```python
from build123d import *

# Parameters (mm, degrees)
SKETCH1_R           = 40.5
SKETCH1_R_2         = 1.75
SKETCH1_R_3         = 33.75
BOSS_EXTRUDE1_DEPTH = 15.5
SKETCH2_R           = 0.75
CUT_EXTRUDE1_DEPTH  = 60.335908184


with BuildPart() as part:
    # Sketch1 → Boss-Extrude1 (new body)
    with BuildSketch(Plane(origin=(0, 0, 0), x_dir=(1, 0, 0), z_dir=(0, 1, 0))):
        with Locations(Location((0, 0, 0), (0, 0, 270))):
            Circle(SKETCH1_R)
        with Locations(Location((0, 37.25, 0), (0, 0, 270))):
            Circle(SKETCH1_R_2, mode=Mode.SUBTRACT)
        with Locations(Location((21.895000648, 30.13588304, 0), (0, 0, 270))):
            Circle(SKETCH1_R_2, mode=Mode.SUBTRACT)
        with Locations(Location((35.426855232, 11.51088304, 0), (0, 0, 270))):
            Circle(SKETCH1_R_2, mode=Mode.SUBTRACT)
        with Locations(Location((35.426855232, -11.51088304, 0), (0, 0, 270))):
            Circle(SKETCH1_R_2, mode=Mode.SUBTRACT)
        with Locations(Location((21.895000648, -30.13588304, 0), (0, 0, 270))):
            Circle(SKETCH1_R_2, mode=Mode.SUBTRACT)
        with Locations(Location((0, -37.25, 0), (0, 0, 270))):
            Circle(SKETCH1_R_2, mode=Mode.SUBTRACT)
        with Locations(Location((-21.895000648, -30.13588304, 0), (0, 0, 270))):
            Circle(SKETCH1_R_2, mode=Mode.SUBTRACT)
        with Locations(Location((-35.426855232, -11.51088304, 0), (0, 0, 270))):
            Circle(SKETCH1_R_2, mode=Mode.SUBTRACT)
        with Locations(Location((-35.426855232, 11.51088304, 0), (0, 0, 270))):
            Circle(SKETCH1_R_2, mode=Mode.SUBTRACT)
        with Locations(Location((-21.895000648, 30.13588304, 0), (0, 0, 270))):
            Circle(SKETCH1_R_2, mode=Mode.SUBTRACT)
        with Locations(Location((0, 0, 0), (0, 0, 270))):
            Circle(SKETCH1_R_3, mode=Mode.SUBTRACT)
    extrude(amount=BOSS_EXTRUDE1_DEPTH)

    # Sketch2 → Cut-Extrude1 (cut, through all)
    with BuildSketch(Plane(origin=(0, 15.5, 0), x_dir=(1, 0, 0), z_dir=(0, 1, 0))):
        with Locations(Location((-6.483486619, -35.325442924, 0), (0, 0, 270))):
            Circle(SKETCH2_R)
        with Locations(Location((-15.518523524, -32.389781477, 0), (0, 0, 270))):
            Circle(SKETCH2_R)
    extrude(amount=-CUT_EXTRUDE1_DEPTH, mode=Mode.SUBTRACT)


solid = part.part
```
Geometry check sheet. Reference: the model listing, model coordinates, mm. Coordinates: 2 decimals unless noted, no trailing zeros. Order: outer loops, then holes, each group sorted by start corner. A loop starts at its lowest first (then second) coordinate and runs counter-clockwise, first axis right, second up.
Q1. Depth check by flat-ended pin: pin 1 Ø4 at (y, z) = (4.5, -11) entering from +X; pin 2 Ø5 at (y, z) = (13, 23.5) entering from +X; pin 3 Ø2 at (x, y) = (24, 5) entering from -Z. Enter the tip coordinate at first touch or a pass-through.
Reply:
pin 1: stops at x = 39.49
pin 2: stops at x = 34.63
pin 3: stops at z = -33.34
Q2. Thickness scan on probe 1 along Z at (x, y) = (23, 3.75); probe 2 along X at (y, z) = (6.5, 0); probe 3 along X at (y, z) = (9, 10). Record the ranges inside material, lowest first.
Reply:
probe 1: z = -33.34 to -31.49, -28.78 to -24.7, 24.7 to 28.78, 31.49 to 33.34
probe 2: x = -40.5 to -33.75, 33.75 to 40.5
probe 3: x = -39.25 to -36.31, -34.54 to -32.23, 32.23 to 34.54, 36.31 to 39.25
Q3. Draft check along Z on faces 1 (the face through (24, 0, -24)), 2 (the face through (21.972, 7.642, -31.884)), 3 (the face through (-0.67, 7.642, 38.867)), 4 (the face through (34.15, 7.64, 21.77)). Enter one of: released by +Z, released by -Z, zero draft, split by the parting line, or undercut.
Reply:
face 1: zero draft
face 2: undercut
face 3: undercut
face 4: split by the parting line
Q4. Sectioned sample at B-B on x = 28. Record the cut outline in (y, z), and give its area (3 significant figures).
Reply:
outline: (0, -29.26) - (15.5, -29.26) - (15.5, -18.84) - (0, -18.84) - close; (0, 18.84) - (15.5, 18.84) - (15.5, 29.26) - (0, 29.26) - close
area: 323 mm2
Q5. Sectioned sample at A-A on z = 0. Record the cut outline in (x, y), and give its area (3 significant figures).
Reply:
outline: (-40.5, 0) - (-33.75, 0) - (-33.75, 15.5) - (-40.5, 15.5) - close; (33.75, 0) - (40.5, 0) - (40.5, 15.5) - (33.75, 15.5) - close
area: 209 mm2
Q6. Sectioned sample at D-D on y = 6.5. Give the number of separate pieces and of enclosed holes in the cut face, and give its area (3 significant figures).
Reply:
separate pieces: 1
enclosed holes: 13
area: 1,470 mm2
Q7. Sectioned sample at C-C on x = 0. Record the cut outline in (y, z), and give its area (3 significant figures).
Reply:
outline: (0, -40.5) - (15.5, -40.5) - (15.5, -39) - (0, -39) - close; (0, -35.5) - (15.5, -35.5) - (15.5, -33.75) - (0, -33.75) - close; (0, 33.75) - (15.5, 33.75) - (15.5, 35.5) - (0, 35.5) - close; (0, 39) - (15.5, 39) - (15.5, 40.5) - (0, 40.5) - close
area: 101 mm2
